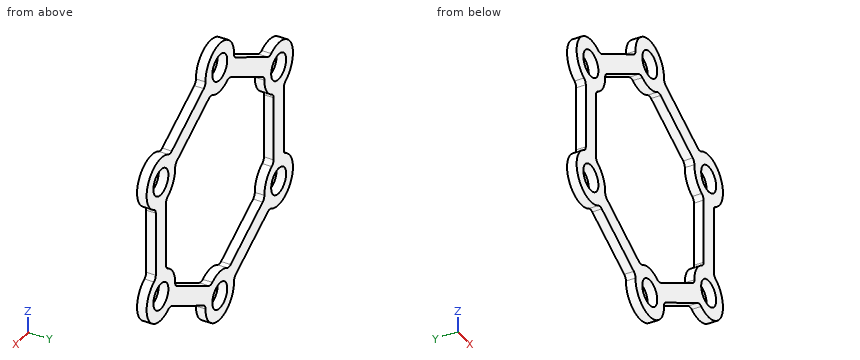
from build123d import *

# Parameters (mm, degrees)
SKETCH2_R           = 2.1
SKETCH2_R_2         = 1.1
BOSS_EXTRUDE1_DEPTH = 0.8
CIRPATTERN1_COUNT   = 6
FILLET1_R           = 0.5


with BuildPart() as part:
    # Sketch2 → Boss-Extrude1 (new body)
    # profile 1 of 2: a face of its own
    with BuildSketch(Plane(origin=(0, 0, 0), x_dir=(1, 0, 0), z_dir=(0, 1, 0))):
        with Locations((0, 10)):
            Circle(SKETCH2_R)
        with Locations(Location((0, 10, 0), (0, 0, 270))):
            Circle(SKETCH2_R_2, mode=Mode.SUBTRACT)
    # profile 2 of 2: a face of its own
    with BuildSketch(Plane(origin=(0, 0, 0), x_dir=(1, 0, 0), z_dir=(0, 1, 0))):
        with BuildLine():
            ThreePointArc((2.073712748, 9.668766791), (1.818653348, 8.95), (1.323712748, 8.369728685))
            Line((1.323712748, 8.369728685), (6.58654129, 5.331233209))
            ThreePointArc((6.58654129, 5.331233209), (6.84160069, 6.05), (7.33654129, 6.630271315))
            Line((7.33654129, 6.630271315), (2.073712748, 9.668766791))
        make_face()
    boss_extrude1 = extrude(amount=BOSS_EXTRUDE1_DEPTH)

    # CirPattern1: Boss-Extrude1 ×6 about axis
    cirpattern1_axis = Axis((0, 0, 0), (0, 1, 0))
    for i in range(1, CIRPATTERN1_COUNT):
        add(boss_extrude1.rotate(cirpattern1_axis, i * 360 / CIRPATTERN1_COUNT))

    # Fillet1
    fillet1_edges = [part.edges().sort_by_distance(p)[0] for p in [
        (2.073712748, 0.4, -9.668766791),
        (7.33654129, 0.4, -6.630271315),
        (6.58654129, 0.4, -5.331233209),
        (1.323712748, 0.4, -8.369728685),
        (9.410254038, 0.4, -3.038495475),
        (7.910254038, 0.4, -3.038495475),
        (9.410254038, 0.4, 3.038495475),
        (7.910254038, 0.4, 3.038495475),
        (7.33654129, 0.4, 6.630271315),
        (6.58654129, 0.4, 5.331233209),
        (2.073712748, 0.4, 9.668766791),
        (1.323712748, 0.4, 8.369728685),
        (-2.073712748, 0.4, 9.668766791),
        (-1.323712748, 0.4, 8.369728685),
        (-7.33654129, 0.4, 6.630271315),
        (-6.58654129, 0.4, 5.331233209),
        (-9.410254038, 0.4, 3.038495475),
        (-7.910254038, 0.4, 3.038495475),
        (-9.410254038, 0.4, -3.038495475),
        (-7.910254038, 0.4, -3.038495475),
        (-7.33654129, 0.4, -6.630271315),
        (-6.58654129, 0.4, -5.331233209),
        (-1.323712748, 0.4, -8.369728685),
        (-2.073712748, 0.4, -9.668766791),
    ]]
    fillet(fillet1_edges, radius=FILLET1_R)


solid = part.part
Geometry: final body of the model. Coordinates: model frame, mm. Give positions to 0.01 mm unless a question says otherwise; leave off trailing zeros. Order: outer loops, then holes, each group sorted by start corner. A loop starts at its lowest first (then second) coordinate and runs counter-clockwise, first axis right, second up. Notation, with made-up numbers: (8, -13.75) -> (18, -13.75) arc R21 ccw to (18, 7.25) -> close; hole circle Ø1 at (-21, 67). An arc over 180 degrees is marked (long way). Answer as a JSON object with one key per item and string values.
Q1. Section A-A (x = 0). Output: boundary loops of the cut face in (y, z).
Entries:
{"outline": "(0, -12.1) -> (0.8, -12.1) -> (0.8, -11.1) -> (0, -11.1) -> close; (0, -8.9) -> (0.8, -8.9) -> (0.8, -7.9) -> (0, -7.9) -> close; (0, 7.9) -> (0.8, 7.9) -> (0.8, 8.9) -> (0, 8.9) -> close; (0, 11.1) -> (0.8, 11.1) -> (0.8, 12.1) -> (0, 12.1) -> close"}
Q2. Section D-D (y = 0.6). State how many separate pieces and enclosed holes the cut face has, plus the area to 3 significant figures.
Entries:
{"separate pieces": "1", "enclosed holes": "7", "area": "114 mm^2"}
Q3. Section C-C (x = -2.75). Output: boundary loops of the cut face in (y, z).
Entries:
{"outline": "(0, -9.28) -> (0.8, -9.28) -> (0.8, -7.55) -> (0, -7.55) -> close; (0, 7.55) -> (0.8, 7.55) -> (0.8, 9.28) -> (0, 9.28) -> close"}
Q4. Section B-B (z = -4.75). Output: boundary loops of the cut face in (x, y), plus the area to 3 significant figures.
Entries:
{"outline": "(-10.75, 0) -> (-9.73, 0) -> (-9.73, 0.8) -> (-10.75, 0.8) -> close; (-7.59, 0) -> (-6.58, 0) -> (-6.58, 0.8) -> (-7.59, 0.8) -> close; (6.58, 0) -> (7.59, 0) -> (7.59, 0.8) -> (6.58, 0.8) -> close; (9.73, 0) -> (10.75, 0) -> (10.75, 0.8) -> (9.73, 0.8) -> close", "area": "3.24 mm^2"}
Q5. Material intervals for probe 1 along X at (y, z) = (0.4, 5); probe 2 along X at (y, z) = (0.6, 10); probe 3 along X at (y, z) = (0.2, -1.75), sorted ascending.
Entries:
{"probe 1": "x = -10.76 to -9.76, -7.56 to -6.56, 6.56 to 7.56, 9.76 to 10.76", "probe 2": "x = -2.1 to -1.1, 1.1 to 2.1", "probe 3": "x = -9.41 to -7.91, 7.91 to 9.41"}
